Could you check a few things on this model? Use its own coordinates, in mm. A direction names the side the tool comes from. Give positions to 0.01 mm unless a question says otherwise; leave off trailing zeros. Order: outer loops, then holes, each group sorted by start corner. A loop starts at its lowest first (then second) coordinate and runs counter-clockwise, first axis right, second up. Notation, with made-up numbers: M 41.25,-9.75 L 57.25,-9.75 A19 ccw 57.25,6.25 Z; hole C -37,45 d9. An arc over 180 degrees is marked long. Answer in a Markdown table with one row per item. Add a question column.
```python
from build123d import *

# Parameters (mm, degrees)
CROQUIS1_W              = 49.8
CROQUIS1_H              = 39.8
CROQUIS1_R              = 2.7
SALIENTE_EXTRUIR1_DEPTH = 6
CORTAR_EXTRUIR1_DEPTH   = 4
REDONDEO1_R             = 3
SALIENTE_EXTRUIR3_DEPTH = 3
CROQUIS5_R              = 6.35
CORTAR_EXTRUIR2_DEPTH   = 3
SALIENTE_EXTRUIR4_DEPTH = 10
SALIENTE_EXTRUIR5_DEPTH = 2
CORTAR_EXTRUIR3_START   = -3
CORTAR_EXTRUIR3_DEPTH   = 3
CORTAR_EXTRUIR4_DEPTH   = 4
CROQUIS10_W             = 4
CROQUIS10_H             = 7
SALIENTE_EXTRUIR6_DEPTH = 4
CORTAR_EXTRUIR5_DEPTH   = 4
CROQUIS16_W             = 28.958796265
CROQUIS16_H             = 47.870649268
CORTAR_EXTRUIR6_DEPTH   = 2
CROQUIS17_W             = 5
CROQUIS17_H             = 16
CORTAR_EXTRUIR7_DEPTH   = 10
CORTAR_EXTRUIR8_DEPTH   = 2
SALIENTE_EXTRUIR7_DEPTH = 10
CROQUIS21_W             = 10
CROQUIS21_H             = 17
SALIENTE_EXTRUIR8_DEPTH = 15
CROQUIS22_R             = 7
CORTAR_EXTRUIR9_DEPTH   = 8
REDONDEO2_R             = 3


with BuildPart() as part:
    # Croquis1 → Saliente-Extruir1 (new body)
    with BuildSketch(Plane.XY):
        with Locations((-31.963412372, -3.757931034)):
            Rectangle(CROQUIS1_W, CROQUIS1_H)
        with Locations((-52.963412372, 12.342068966)):
            Circle(CROQUIS1_R, mode=Mode.SUBTRACT)
        with Locations((-10.963412372, 12.342068966)):
            Circle(CROQUIS1_R, mode=Mode.SUBTRACT)
        with Locations((-10.963412372, -19.657931034)):
            Circle(CROQUIS1_R, mode=Mode.SUBTRACT)
        with Locations((-52.963412372, -19.657931034)):
            Circle(CROQUIS1_R, mode=Mode.SUBTRACT)
    extrude(amount=SALIENTE_EXTRUIR1_DEPTH)

    # Croquis2 → Cortar-Extruir1 (cut)
    with BuildSketch(Plane.XY.offset(6)):
        with BuildLine():
            Line((-49.963412372, -16.757931034), (-13.963412372, -16.757931034))
            ThreePointArc((-13.963412372, -16.757931034), (-12.54919881, -16.172144597), (-11.963412372, -14.757931034))
            Line((-11.963412372, -14.757931034), (-11.963412372, 7.242068966))
            ThreePointArc((-11.963412372, 7.242068966), (-12.54919881, 8.656282528), (-13.963412372, 9.242068966))
            Line((-13.963412372, 9.242068966), (-49.963412372, 9.242068966))
            ThreePointArc((-49.963412372, 9.242068966), (-51.377625934, 8.656282528), (-51.963412372, 7.242068966))
            Line((-51.963412372, 7.242068966), (-51.963412372, -14.757931034))
            ThreePointArc((-51.963412372, -14.757931034), (-51.377625934, -16.172144597), (-49.963412372, -16.757931034))
        make_face()
    extrude(amount=-CORTAR_EXTRUIR1_DEPTH, mode=Mode.SUBTRACT)

    # Redondeo1
    redondeo1_edges = [part.edges().sort_by_distance(p)[0] for p in [
        (-56.863412372, 16.142068966, 3),
        (-7.063412372, 16.142068966, 3),
        (-7.063412372, -23.657931034, 3),
        (-56.863412372, -23.657931034, 3),
    ]]
    fillet(redondeo1_edges, radius=REDONDEO1_R)

    # Croquis4 → Saliente-Extruir3 (add)
    with BuildSketch(Plane(origin=(0, 0, 0), x_dir=(-1, 0, 0), z_dir=(0, 0, -1))):
        with BuildLine():
            Line((56.863412372, 4.242068966), (61.863412372, 4.242068966))
            Line((61.863412372, 4.242068966), (61.863412372, -0.257931034))
            Line((61.863412372, -0.257931034), (57.863412372, -0.257931034))
            ThreePointArc((57.863412372, -0.257931034), (57.358118834, -0.294597605), (56.863412372, -0.403829068))
            Line((56.863412372, -0.403829068), (56.863412372, 4.242068966))
        make_face()
        with BuildLine():
            Line((61.863412372, -11.757931034), (56.863412372, -11.757931034))
            Line((56.863412372, -11.757931034), (56.863412372, -7.112033001))
            ThreePointArc((56.863412372, -7.112033001), (57.358118834, -7.221264464), (57.863412372, -7.257931034))
            Line((57.863412372, -7.257931034), (61.863412372, -7.257931034))
            Line((61.863412372, -7.257931034), (61.863412372, -11.757931034))
        make_face()
    extrude(amount=-SALIENTE_EXTRUIR3_DEPTH)

    # Croquis5 → Cortar-Extruir2 (cut)
    with BuildSketch(Plane.XY.offset(3)):
        with Locations((-57.863412372, -3.757931034)):
            Circle(CROQUIS5_R)
    extrude(amount=CORTAR_EXTRUIR2_DEPTH, mode=Mode.SUBTRACT)

    # Croquis6 → Saliente-Extruir4 (add)
    with BuildSketch(Plane.XY.offset(3)):
        with BuildLine():
            Line((-61.863412372, 4.242068966), (-51.963412372, 4.242068966))
            Line((-51.963412372, 4.242068966), (-48.963412372, 4.242068966))
            Line((-48.963412372, 4.242068966), (-48.963412372, -11.757931034))
            Line((-48.963412372, -11.757931034), (-51.963412372, -11.757931034))
            Line((-51.963412372, -11.757931034), (-61.863412372, -11.757931034))
            Line((-61.863412372, -11.757931034), (-61.863412372, -8.689715701))
            ThreePointArc((-61.863412372, -8.689715701), (-51.513412372, -3.757931034), (-61.863412372, 1.173853632))
            Line((-61.863412372, 1.173853632), (-61.863412372, 4.242068966))
        make_face()
    extrude(amount=SALIENTE_EXTRUIR4_DEPTH)

    # Croquis7 → Saliente-Extruir5 (add)
    with BuildSketch(Plane.XY.offset(2)):
        Polygon((-51.963412372, -3.757931034), (-51.963412372, 4.242068966), (-48.963412372, 4.242068966), (-48.963412372, -11.757931034), (-51.963412372, -11.757931034), align=None)
    extrude(amount=SALIENTE_EXTRUIR5_DEPTH)

    # Croquis8 → Cortar-Extruir3 (cut)
    with BuildSketch(Plane.XY.offset(3).offset(CORTAR_EXTRUIR3_START)):
        with BuildLine():
            Line((-56.863412372, -0.403829068), (-56.863412372, -7.112033001))
            ThreePointArc((-56.863412372, -7.112033001), (-53.509310406, -3.757931034), (-56.863412372, -0.403829068))
        make_face()
    extrude(amount=CORTAR_EXTRUIR3_DEPTH, mode=Mode.SUBTRACT)

    # Croquis9 → Cortar-Extruir4 (cut)
    with BuildSketch(Plane.XY.offset(6)):
        Polygon((-56.863412372, -11.757931034), (-56.863412372, -27.492217147), (-1.817084798, -27.492217147), (-1.817084798, 22.861833321), (-56.863412372, 22.861833321), (-56.863412372, 4.242068966), (-47.172737702, 4.242068966), (-47.172737702, -11.757931034), align=None)
    extrude(amount=-CORTAR_EXTRUIR4_DEPTH, mode=Mode.SUBTRACT)

    # Croquis10 → Saliente-Extruir6 (add)
    with BuildSketch(Plane.XY.offset(2)):
        with Locations((-9.063412372, 5.842068966)):
            Rectangle(CROQUIS10_W, CROQUIS10_H)
    extrude(amount=SALIENTE_EXTRUIR6_DEPTH)

    # Croquis11 → Cortar-Extruir5 (cut)
    with BuildSketch(Plane(origin=(-7.063412372, 0, 0), x_dir=(0, 0, -1), z_dir=(1, 0, 0))):
        Polygon((-2, 5.842068966), (-2, 7.242068966), (-4, 7.242068966), (-4, 4.442068966), (-2, 4.442068966), align=None)
    extrude(amount=-CORTAR_EXTRUIR5_DEPTH, mode=Mode.SUBTRACT)

    # Croquis16 → Cortar-Extruir6 (cut)
    with BuildSketch(Plane.XY.offset(2)):
        with Locations((-49.718694927, -6.990346687)):
            Rectangle(CROQUIS16_W, CROQUIS16_H)
    extrude(amount=CORTAR_EXTRUIR6_DEPTH, mode=Mode.SUBTRACT)


with BuildPart() as cortar_extruir6_kept_piece:
    # of the separate pieces the step leaves, the one the design keeps (cortar_extruir6_pieces_kept)
    add(part.part.solids().sort_by_distance((-53.863412372, 16.142068966, 0))[0])

    # Croquis17 → Cortar-Extruir7 (cut)
    with BuildSketch(Plane.XY.offset(2)):
        with Locations((-59.363412372, -3.757931034)):
            Rectangle(CROQUIS17_W, CROQUIS17_H)
    extrude(amount=-CORTAR_EXTRUIR7_DEPTH, mode=Mode.SUBTRACT)

    # Croquis18 → Cortar-Extruir8 (cut)
    with BuildSketch(Plane.XY.offset(2)):
        with BuildLine():
            Line((-56.863412372, -0.403829068), (-50.513412372, -0.403829068))
            ThreePointArc((-50.513412372, -0.403829068), (-47.159310406, -3.757931034), (-50.513412372, -7.112033001))
            Line((-50.513412372, -7.112033001), (-56.863412372, -7.112033001))
            Line((-56.863412372, -7.112033001), (-56.863412372, -0.403829068))
        make_face()
    extrude(amount=-CORTAR_EXTRUIR8_DEPTH, mode=Mode.SUBTRACT)

    # Croquis19 → Saliente-Extruir7 (add)
    with BuildSketch(Plane.XY.offset(2)):
        with BuildLine():
            Line((-56.863412372, -0.403829068), (-55.905304433, -0.403829068))
            ThreePointArc((-55.905304433, -0.403829068), (-48.769281441, 2.347845517), (-44.163412372, -3.757931034))
            ThreePointArc((-44.163412372, -3.757931034), (-48.769281441, -9.863707586), (-55.905304433, -7.112033001))
            Line((-55.905304433, -7.112033001), (-56.863412372, -7.112033001))
            Line((-56.863412372, -7.112033001), (-56.863412372, -10.112033001))
            ThreePointArc((-56.863412372, -10.112033001), (-41.523253228, -3.757931034), (-56.863412372, 2.596170932))
            Line((-56.863412372, 2.596170932), (-56.863412372, -0.403829068))
        make_face()
    extrude(amount=SALIENTE_EXTRUIR7_DEPTH)

    # Croquis21 → Saliente-Extruir8 (add)
    with BuildSketch(Plane.XY.offset(2)):
        with Locations((-24.063412372, 7.642068966)):
            Rectangle(CROQUIS21_W, CROQUIS21_H)
    extrude(amount=SALIENTE_EXTRUIR8_DEPTH)

    # Croquis22 → Cortar-Extruir9 (cut)
    with BuildSketch(Plane.ZY.offset(29.063412372)):
        with Locations(Location((9, 7.642068966, 0), (0, 0, 270))):
            Circle(CROQUIS22_R)
    extrude(amount=-CORTAR_EXTRUIR9_DEPTH, mode=Mode.SUBTRACT)

    # Redondeo2
    redondeo2_edges = [cortar_extruir6_kept_piece.edges().sort_by_distance(p)[0] for p in [
        (-24.063412372, 16.142068966, 17),
        (-24.063412372, -0.857931034, 17),
    ]]
    fillet(redondeo2_edges, radius=REDONDEO2_R)


solid = cortar_extruir6_kept_piece.part
```
1. For faces 1 (the cylindrical face through (-41.53, -4.05, 6.93)), 2 (the flat face through (-9, 6, 4)), 3 (the flat face through (-9, 9.342, 4)), 4 (the flat face through (-29.063, 6, 16)), 5 (the flat face through (-9, 6, 6)), which set-ups out of +Z, -Z, +X, -X, +Y, -Y let a thin tool reach every point of the face, with its end or its side?
2. Suppose I cut it at C-C on z = 9. List the corners of the cut face in (x, y) for me.
3. Thinking about a two-plate mould opening in Y: for faces 6 (the flat face through (-56.863, -9, 3)), 7 (the cylindrical face through (-9.512, -17.381, 0.986)), 8 (the cylindrical face through (-7.966, -22.802, 1.014)), which applies, pulls with the +Y half, pulls with the -Y half, needs draft (parallel to the pull), parting line crosses it, or undercut?
4. Suppose I cut it at B-B on z = 4.75. List the corners of the cut face in (x, y) for me.
5. Will these pins go through, and if not, where does the flat tip stop? P1, Ø3, axis at x = -26, z = 6.5, coming from the -Y side; P2, Ø0.8, axis at x = -9, y = 6.5, coming from the -Z side; P3, Ø1.9, axis at x = -52.5, z = 5.5, coming from the -Y side; P4, Ø4.5, axis at y = 6.5, z = 5, coming from the -X side.
6. Suppose I cut it at A-A on x = -27. List the corners of the cut face in (y, z) for me.
7. Suppose I cut it at D-D on y = -9.5. List the corners of the cut face in (x, z) for me.
8. If I drill on line 1 along X through (y, z) = (0, 7.25); line 2 along Y through (x, z) = (-10, 2.5); line 3 along X through (y, z) = (14, 3.5), over which ranges is the centre line in solid material (lowest first)? Write a range as [from, to].
Findings below:
| question | item | result |
|---|---|---|
| 1 | face 1 | +Z |
| 1 | face 2 | +X |
| 1 | face 3 | +Z, +X, +Y |
| 1 | face 4 | +Z, +Y, -Y |
| 1 | face 5 | +Z, +X, +Y, -Y |
| 2 | outline | M -56.86,-10.11 A8.99 ccw long -56.86,2.6 L -56.86,-0.4 L -55.91,-0.4 A6.35 cw long -55.91,-7.11 L -56.86,-7.11 Z; M -29.06,-0.86 L -19.06,-0.86 L -19.06,16.14 L -29.06,16.14 L -29.06,14.64 L -21.06,14.64 L -21.06,0.64 L -29.06,0.64 Z |
| 3 | face 6 | needs draft |
| 3 | face 7 | undercut |
| 3 | face 8 | pulls with the -Y half |
| 4 | outline | M -56.86,-10.11 A8.99 ccw long -56.86,2.6 L -56.86,-0.4 L -55.91,-0.4 A6.35 cw long -55.91,-7.11 L -56.86,-7.11 Z; M -29.06,-0.86 L -19.06,-0.86 L -19.06,16.14 L -29.06,16.14 L -29.06,13.2 L -21.06,13.2 L -21.06,2.08 L -29.06,2.08 Z; M -11.06,2.34 L -7.06,2.34 L -7.06,9.34 L -11.06,9.34 Z |
| 5 | P1 | y = -0.86 |
| 5 | P2 | z = 0 |
| 5 | P3 | y = -12.68 |
| 5 | P4 | x = -54.59 |
| 6 | outline | M -23.66,0 L 16.14,0 L 16.14,14 A3 ccw 13.14,17 L 2.14,17 A3 ccw -0.86,14 L -0.86,2 L -23.66,2 Z; hole C 7.64,9 d14 |
| 7 | outline | M -56.86,0 L -7.06,0 L -7.06,2 L -43.6,2 L -43.6,12 L -47.8,12 L -47.8,2 L -53.22,2 L -53.22,12 L -56.86,12 Z |
| 8 | line 1 | [-56.86, -55.63], [-45.39, -42.35], [-29.06, -19.06] |
| 8 | line 2 | [2.34, 4.44], [7.24, 9.34] |
| 8 | line 3 | [-29.06, -19.06] |
